Drawing for the job (mm, zero at the part's lowest x, y, z). A direction names the side the tool comes from. Coordinates: 2 decimals unless noted, no trailing zeros. Order: outer loops, then holes, each group sorted by start corner. A loop starts at its lowest first (then second) coordinate and runs counter-clockwise, first axis right, second up. Notation, with made-up numbers: (25.25, -14.5) - (84.25, -14.5) arc R33 ccw to (84.25, 21.5) - close; hole circle Ø8 at (-16, 28). An arc over 180 degrees is marked (long way). Put each result on its own line as item: value. Start each with the question number.
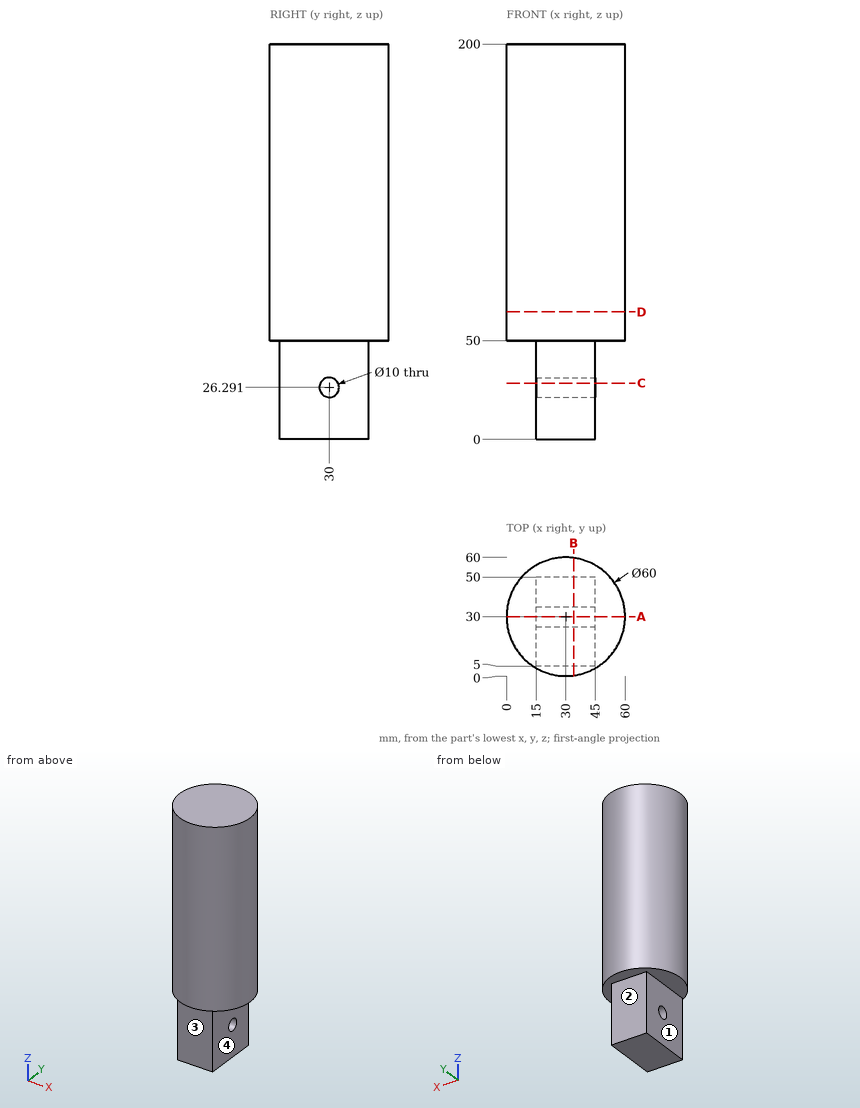
Item 1: Slice it at A-A, the plane y = 30. Give the cut face in (x, z).
Item 2: Flat gauge pins, fed straight in: pin 1 Ø11.5 at (y, z) = (30, 26.29) entering from -X; pin 2 Ø1 at (x, y) = (53, 35) entering from -Z; pin 3 Ø6 at (y, z) = (22.5, 38.5) entering from +X. Where does each tip first touch, or does it go through?
Item 3: Wall check: line 1 along Z through (x, y) = (32.25, 30); line 2 along Y through (x, z) = (20, 15); line 3 along Z through (x, y) = (10, 11). Give the ranges that are in metal, low to high.
Item 4: Slice it at C-C, the plane z = 28.5. Give the cut face in (x, y), plus the area to 3 significant figures.
Item 5: Slice it at B-B, the plane x = 34. Give the cut face in (y, z), plus the area to 3 significant figures.
Item 6: Slice it at D-D, the plane z = 64.5. Give the cut face in (x, y).
Item 7: 3-axis set-ups, long thin cutter, end or side, ignore diameter. For the marked faces 1, 2, 3 and 4: which of +Z, -Z, +X, -X, +Y, -Y reach the whole face in a straight line?
Here are the results:
1. outline: (0, 50) - (15, 50) - (15, 31.29) - (45, 31.29) - (45, 50) - (60, 50) - (60, 200) - (0, 200) - close; (15, 0) - (45, 0) - (45, 21.29) - (15, 21.29) - close
2. pin 1: stops at x = 15
2. pin 2: stops at z = 50
2. pin 3: stops at x = 45
3. line 1: z = 0 to 21.29, 31.29 to 200
3. line 2: y = 5 to 50
3. line 3: z = 50 to 200
4. outline: (15, 5) - (45, 5) - (45, 25.51) - (15, 25.51) - close; (15, 34.49) - (45, 34.49) - (45, 50) - (15, 50) - close
4. area: 1,080 mm^2
5. outline: (0.27, 50) - (5, 50) - (5, 0) - (50, 0) - (50, 50) - (59.73, 50) - (59.73, 200) - (0.27, 200) - close; hole circle Ø10 at (30, 26.29)
5. area: 11,100 mm^2
6. outline: circle Ø60 at (30, 30)
7. face 1: -Z, -X, +Y, -Y
7. face 2: -Z, +X, -X, +Y
7. face 3: -Z, +X, -X, -Y
7. face 4: -Z, +X, +Y, -Y
